from build123d import *


with BuildPart() as f3:
    # F0 (on Top) → F3 section 0
    with BuildSketch(Plane.XY, mode=Mode.PRIVATE) as f3_s0:
        Polygon((20.656764, 73.207314), (-37.295084, 65.84017), (-73.063872, 19.652667), (-65.696728, -38.299182), (-19.509226, -74.067969), (38.442623, -66.700826), (74.211411, -20.513323), (66.844267, 37.438526), align=None)
    loft([Vertex(0.573766, 0.007616, 100), f3_s0.sketch])


solid = f3.part
CAD build for the part. Positions are in the model's coordinates, mm. Coordinates: 2 decimals unless noted, no trailing zeros. Loops run counter-clockwise (first coordinate to the right, second up) from the corner with the lowest first, then second, coordinate; pieces in that order, holes last. Notation, with made-up numbers: (55, 54) - (102, 54) arc R19 ccw to (102, 66) - close; hole circle Ø3 at (13.5, -14.5). An arc over 180 degrees is marked (long way). Write item = value, one per line. Start each with the question number.
Q1. Cut at B-B, the plane x = 7.5. List the corners of the cut face in (y, z), then the cut area to 3 significant figures.
Q2. Cut at A-A, the plane z = 26. List the corners of the cut face in (x, y).
Q3. Flat gauge pins, fed straight in: pin 1 Ø5 at (x, y) = (14.5, -19) entering from -Z; pin 2 Ø6 at (x, z) = (-3, 35) entering from -Y; pin 3 Ø12 at (x, y) = (-18.5, -12.5) entering from +Z; pin 4 Ø10 at (x, z) = (-0.5, 14.5) entering from -Y. Where does each tip first touch, or does it go through?
Q4. Drill centre lines: L1, parallel to Z at x = -43, y = 5.5; L2, parallel to Z at x = -20, y = 62; L3, parallel to X at y = 8, z = 61. Where is each one in solid material? Low to high.
Q5. Cut at C-C, the plane y = 9.5. List the corners of the cut face in (x, z).
Q6. Cut at D-D, the plane z = 67.5. List the corners of the cut face in (x, y), then the cut area to 3 significant figures.
Computed:
q1.outline = (-70.63, 0) - (71.53, 0) - (25.25, 65.51) - (3.92, 89.55) - (-1.92, 90.59) - (-12.19, 81.71) - close
q1.area = 6,970 mm²
q2.outline = (-53.92, 14.54) - (-48.47, -28.34) - (-14.29, -54.81) - (28.6, -49.36) - (55.07, -15.18) - (49.61, 27.71) - (15.44, 54.18) - (-27.45, 48.72) - close
q3.pin_1 = 0
q3.pin_2 = -49.12
q3.pin_3 = 77.91
q3.pin_4 = -64.91
q4.L1 = 0 to 39.73
q4.L2 = 0 to 8.55
q4.L3 = -27.89 to 27.26
q5.outline = (-71.77, 0) - (70.4, 0) - (17.38, 74.64) - (3.18, 87.03) - (-4.89, 85.58) - (-35.01, 51.68) - close
q6.outline = (-23.36, 6.39) - (-20.96, -12.44) - (-5.95, -24.07) - (12.88, -21.67) - (24.51, -6.66) - (22.11, 12.17) - (7.1, 23.8) - (-11.73, 21.4) - close
q6.area = 1,740 mm²
